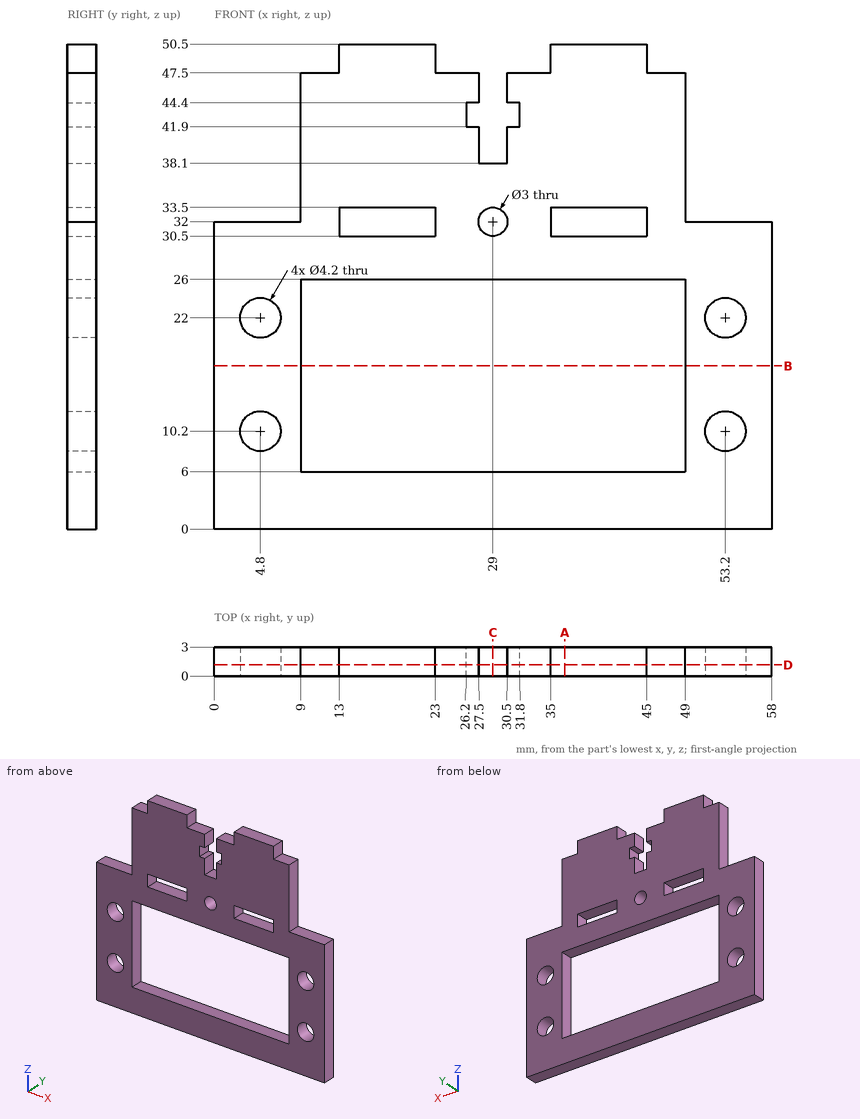
Part print with two shaded views. Sizes in mm from the minimum x, y, z corner. Round coordinates to 2 decimals unless told otherwise and drop trailing zeros. Write each loop counter-clockwise with the first axis right and the second up, starting at its lowest first coordinate (ties: lowest second). Pieces come first, ordered by that corner, then holes. Notation, with made-up numbers: M 54,-37 L 107,-37 A22 ccw 107,0 Z; hole C 63.25,16.5 d5. An arc over 180 degrees is marked long. Use CSV: the item, a comma, the result in double quotes.
1. Saw through at B-B (z = 17). Give the cut face in (x, y).
Reply:
outline,"M 0,0 L 9,0 L 9,3 L 0,3 Z; M 49,0 L 58,0 L 58,3 L 49,3 Z"
2. Saw through at D-D (y = 1.15). State how many separate pieces and enclosed holes the cut face has, plus the area to 3 significant figures.
Reply:
separate pieces,"1"
enclosed holes,"8"
area,"1,580 mm²"
3. Saw through at A-A (x = 36.5). Give the cut face in (y, z), plus the area to 3 significant figures.
Reply:
outline,"M 0,0 L 3,0 L 3,6 L 0,6 Z; M 0,26 L 3,26 L 3,30.5 L 0,30.5 Z; M 0,33.5 L 3,33.5 L 3,50.5 L 0,50.5 Z"
area,"82.5 mm²"
4. Saw through at C-C (x = 29). Give the cut face in (y, z), plus the area to 3 significant figures.
Reply:
outline,"M 0,0 L 3,0 L 3,6 L 0,6 Z; M 0,26 L 3,26 L 3,30.5 L 0,30.5 Z; M 0,33.5 L 3,33.5 L 3,38.1 L 0,38.1 Z"
area,"45.3 mm²"
5. Wall check: probe 1 along Z at (x, y) = (41.5, 2.45); probe 2 along X at (y, z) = (0.6, 22); probe 3 along X at (y, z) = (1.7, 48.5). Give the ranges that are in metal, low to high. Write a range as from..to.
Reply:
probe 1,"z = 0..6, 26..30.5, 33.5..50.5"
probe 2,"x = 0..2.7, 6.9..9, 49..51.1, 55.3..58"
probe 3,"x = 13..23, 35..45"
6. Flat gauge pins, fed straight in: pin 1 (0.7 mm diameter, centred on x = 31, y = 2, fed in from -Z); pin 2 (1.5 mm diameter, centred on x = 25.5, y = 2, fed in from +Z); pin 3 (0.9 mm diameter, centred on y = 1, z = 39.5, fed in from -X); pin 4 (1.5 mm diameter, centred on y = 1, z = 40.5, fed in from +X). Where does each tip first touch, or does it go through?
Reply:
pin 1,"stops at z = 0"
pin 2,"stops at z = 47.5"
pin 3,"stops at x = 9"
pin 4,"stops at x = 49"
